from build123d import *

# Parameters (mm, degrees)
F0_R     = 8.25
F1_DEPTH = 1
F2_R     = 7
F3_DEPTH = 25
F5_DEPTH = 5


with BuildPart() as f1:
    # F0 (on Front) → F1 (new body)
    with BuildSketch(Plane.XZ):
        Circle(F0_R)
    extrude(amount=F1_DEPTH)

    # F2 (on Front) → F3 (join)
    with BuildSketch(Plane.XZ):
        Circle(F2_R)
    extrude(amount=F3_DEPTH)

    # F4 (on Top) → F5 (join, symmetric)
    with BuildSketch(Plane.XY):
        with BuildLine():
            ThreePointArc((-4, 4.1967689234), (-5.329329795, 2.2827863089), (-5.7976606831, 0))
            Line((-5.7976606831, 0), (5, 0))
            Line((5, 0), (-4, 4.1967689234))
        make_face()
    extrude(amount=F5_DEPTH, both=True)


solid = f1.part
Build history of the part. All positions in model axes, mm. A direction names the side the tool comes from. Round coordinates to 2 decimals unless told otherwise and drop trailing zeros. Write each loop counter-clockwise with the first axis right and the second up, starting at its lowest first coordinate (ties: lowest second). Pieces come first, ordered by that corner, then holes. Notation, with made-up numbers: (-24.75, 49.5) -> (-19.75, 49.5) arc R22 ccw to (-19.75, 83.5) -> close; hole circle Ø6 at (23.25, 0). An arc over 180 degrees is marked (long way). Use one line per item in the form item = value.
Q1. Drop flat-ended pins along their axis: P1, Ø5, axis at x = 4.5, y = -19.5, coming from the -Z side; P2, Ø6, axis at y = -11.5, z = -1, coming from the -X side; P3, Ø1, axis at y = -17.5, z = -6.5, coming from the -X side. Give the stop position or say it passes through.
Conclusion:
P1 = -6.71
P2 = -7
P3 = -3.61
Q2. Band-saw the part on C-C, the plane y = -20.5. Write the cut outline in (x, z).
Conclusion:
outline = circle Ø14 at (0, 0)
Q3. Drill centre lines: L1, parallel to Y at x = -2.5, z = -5.5; L2, parallel to Z at x = -2.25, y = 1; L3, parallel to Y at x = 6.25, z = -5. Where is each one in solid material? Low to high.
Conclusion:
L1 = -25 to 0
L2 = -5 to 5
L3 = -1 to 0
Q4. Band-saw the part on A-A, the plane z = 0. Write the cut outline in (x, y).
Conclusion:
outline = (-8.25, -1) -> (-7, -1) -> (-7, -25) -> (7, -25) -> (7, -1) -> (8.25, -1) -> (8.25, 0) -> (5, 0) -> (-4, 4.2) arc R5.8 ccw to (-5.8, 0) -> (-8.25, 0) -> close
Q5. Band-saw the part on D-D, the plane x = -6.5. Write the cut outline in (y, z).
Conclusion:
outline = (-25, -2.6) -> (-1, -2.6) -> (-1, -5.08) -> (0, -5.08) -> (0, 5.08) -> (-1, 5.08) -> (-1, 2.6) -> (-25, 2.6) -> close
Q6. Tool access for faces 1 (the flat face through (0.56, 2.07, 0.07)), 2 (the flat face through (-4, -1, -6)), 3 (the flat face through (-2, 2, -5)), 4 (the flat face through (-2, 2, 5)): list every direction of +Z, -Z, +X, -X, +Y, -Y with a clear straight run to the whole face (end or side of a thin tool).
Conclusion:
face_1 = +Z, -Z, +X, +Y
face_2 = -Y
face_3 = -Z, +X, -X, +Y
face_4 = +Z, +X, -X, +Y
Q7. Band-saw the part on B-B, the plane x = -3.25. Write the cut outline in (y, z).
Conclusion:
outline = (-25, -6.2) -> (-1, -6.2) -> (-1, -7.58) -> (0, -7.58) -> (0, -5) -> (3.85, -5) -> (3.85, 5) -> (0, 5) -> (0, 7.58) -> (-1, 7.58) -> (-1, 6.2) -> (-25, 6.2) -> close
